Source: three-view drawing plus pictorial views. Frame: mm from the lowest corner of the part. Give positions to 0.01 mm unless a question says otherwise; leave off trailing zeros. Loops run counter-clockwise (first coordinate to the right, second up) from the corner with the lowest first, then second, coordinate; pieces in that order, holes last. Notation, with made-up numbers: (71.25, 25.5) - (87.25, 25.5) arc R22 ccw to (87.25, 49.5) - close; hole circle Ø8 at (44, 60). An arc over 180 degrees is marked (long way). Answer as a JSON object with one key per item and string values.
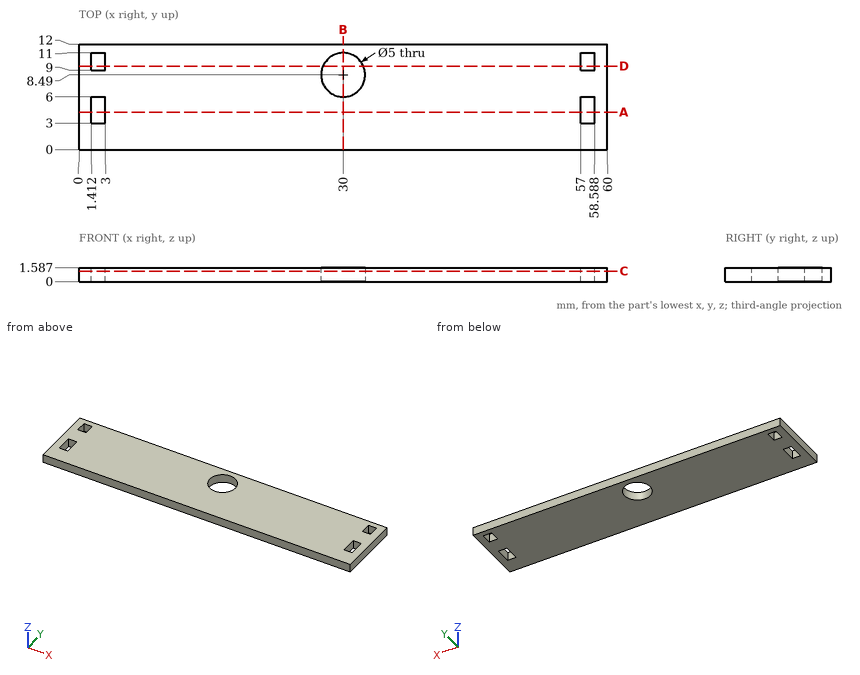
Item 1: Contact query for a flat-ended pin moving along its axis: P1, Ø4, axis at x = 30, y = 8.49, coming from the +Z side. Output: stop coordinate, or through.
Geometry check:
{"P1": "passes through"}
Item 2: Material intervals for line 1 (X direction, y = 5, z = 0.2); line 2 (X direction, y = 8.5, z = 0.5); line 3 (Y direction, x = 30, z = 0.7), sorted ascending. Write a range as [from, to].
Geometry check:
{"line 1": "x = [0, 1.41], [3, 57], [58.59, 60]", "line 2": "x = [0, 27.5], [32.5, 60]", "line 3": "y = [0, 5.99], [10.99, 12]"}
Item 3: Cut plane D-D (y = 9.5). Return loops of the section in (x, z).
Geometry check:
{"outline": "(0, 0) - (1.41, 0) - (1.41, 1.59) - (0, 1.59) - close; (3, 0) - (27.71, 0) - (27.71, 1.59) - (3, 1.59) - close; (32.29, 0) - (57, 0) - (57, 1.59) - (32.29, 1.59) - close; (58.59, 0) - (60, 0) - (60, 1.59) - (58.59, 1.59) - close"}
Item 4: Cut plane A-A (y = 4.25). Return loops of the section in (x, z).
Geometry check:
{"outline": "(0, 0) - (1.41, 0) - (1.41, 1.59) - (0, 1.59) - close; (3, 0) - (57, 0) - (57, 1.59) - (3, 1.59) - close; (58.59, 0) - (60, 0) - (60, 1.59) - (58.59, 1.59) - close"}
Item 5: Cut plane B-B (x = 30). Return loops of the section in (y, z), then the cut area to 3 significant figures.
Geometry check:
{"outline": "(0, 0) - (5.99, 0) - (5.99, 1.59) - (0, 1.59) - close; (10.99, 0) - (12, 0) - (12, 1.59) - (10.99, 1.59) - close", "area": "11.1 mm2"}
Item 6: Cut plane C-C (z = 1.2). Return loops of the section in (x, y).
Geometry check:
{"outline": "(0, 0) - (60, 0) - (60, 12) - (0, 12) - close; hole (1.41, 3) - (3, 3) - (3, 6) - (1.41, 6) - close; hole (1.41, 9) - (3, 9) - (3, 11) - (1.41, 11) - close; hole circle Ø5 at (30, 8.49); hole (57, 3) - (58.59, 3) - (58.59, 6) - (57, 6) - close; hole (57, 9) - (58.59, 9) - (58.59, 11) - (57, 11) - close"}
